The model under review builds one solid part; all positions refer to its coordinate system, in mm. A direction names the side the tool comes from. Give positions to 0.01 mm unless a question says otherwise; leave off trailing zeros. Order: outer loops, then holes, each group sorted by start corner. A loop starts at its lowest first (then second) coordinate and runs counter-clockwise, first axis right, second up.
```python
from build123d import *

# Parameters (mm, degrees)
BOSS_EXTRUDE1_DEPTH              = 5
FILLET1_R                        = 3
TAP_DRILL_FOR_M8X1_25_TAP1_D     = 6.8
TAP_DRILL_FOR_M8X1_25_TAP1_DEPTH = 8
TAP_DRILL_FOR_M8X1_25_TAP1_TIP   = 2.042926105


with BuildPart() as part:
    # Sketch1 → Boss-Extrude1 (new body)
    with BuildSketch(Plane(origin=(0, 0, 0), x_dir=(1, 0, 0), z_dir=(0, 1, 0))):
        with BuildLine():
            Line((32, 42), (-32, 42))
            ThreePointArc((-32, 42), (-39.071067812, 39.071067812), (-42, 32))
            Line((-42, 32), (-42, -32))
            ThreePointArc((-42, -32), (-39.071067812, -39.071067812), (-32, -42))
            Line((-32, -42), (32, -42))
            ThreePointArc((32, -42), (39.071067812, -39.071067812), (42, -32))
            Line((42, -32), (42, 32))
            ThreePointArc((42, 32), (39.071067812, 39.071067812), (32, 42))
        make_face()
    extrude(amount=BOSS_EXTRUDE1_DEPTH)

    # Sketch3 → Revolve2 (revolve)
    with BuildSketch(Plane.XY, mode=Mode.PRIVATE) as revolve2_sk:
        with BuildLine():
            Line((-21.830169384, 5), (-12.5, 5))
            Line((-12.5, 5), (-11.15, 5))
            Line((-11.15, 5), (-11.15, 12))
            Line((-11.15, 12), (-12.5, 12))
            ThreePointArc((-12.5, 12), (-16.03878275, 6.998773158), (-21.830169384, 5))
        make_face()
        with BuildLine():
            Line((-12.5, 12), (-11.15, 12))
            ThreePointArc((-11.15, 12), (-11.537197996, 13.009021804), (-12.5, 13.5))
            Line((-12.5, 13.5), (-15.5, 13.5))
            ThreePointArc((-15.5, 13.5), (-13.822949017, 13.104101966), (-12.5, 12))
        make_face()
    revolve(revolve2_sk.sketch.rotate(Axis((0, 0, 0), (0, -1, 0)), 270), axis=Axis((0, 0, 0), (0, -1, 0)))

    # Sketch3_5 → Cut-Revolve2 (revolve, cut)
    with BuildSketch(Plane.XY, mode=Mode.PRIVATE) as cut_revolve2_sk:
        with BuildLine():
            Line((0, 0), (0, 5))
            Line((0, 5), (-7.6, 5))
            ThreePointArc((-7.6, 5), (-8.694616444, 4.701278719), (-9.6, 4.017392631))
            Line((-9.6, 4.017392631), (-9.6, 0))
            Line((-9.6, 0), (0, 0))
        make_face()
    revolve(cut_revolve2_sk.sketch.rotate(Axis((0, 0, 0), (0, -1, 0)), 270), axis=Axis((0, 0, 0), (0, -1, 0)), mode=Mode.SUBTRACT)

    # Fillet1
    fillet1_edges = [part.edges().sort_by_distance(p)[0] for p in [
        (39.071067812, 5, 39.071067812),
        (0, 5, 42),
        (-39.071067812, 5, 39.071067812),
        (-42, 5, 0),
        (-39.071067812, 5, -39.071067812),
        (0, 5, -42),
        (39.071067812, 5, -39.071067812),
        (42, 5, 0),
    ]]
    fillet(fillet1_edges, radius=FILLET1_R)

    # Tap Drill for M8x1.25 Tap1
    with Locations(Plane(origin=(0, 5, 0), x_dir=(1, 0, 0), z_dir=(0, 1, 0))):
        with Locations((-32, 32), (-32, -32), (32, -32), (32, 32)):
            Hole(TAP_DRILL_FOR_M8X1_25_TAP1_D / 2, depth=TAP_DRILL_FOR_M8X1_25_TAP1_DEPTH)
            with Locations((0, 0, -(TAP_DRILL_FOR_M8X1_25_TAP1_DEPTH + TAP_DRILL_FOR_M8X1_25_TAP1_TIP / 2))):  # 118° drill point
                Cone(0, TAP_DRILL_FOR_M8X1_25_TAP1_D / 2, TAP_DRILL_FOR_M8X1_25_TAP1_TIP, mode=Mode.SUBTRACT)


solid = part.part
```
Item 1: Take a section at A-A (x = 0). Give the boundary of the cut face in (y, z), and give its area (3 significant figures).
Values found:
outline: (0, -42) - (2, -42) arc R3 ccw to (5, -39) - (5, -21.83) arc R10 cw to (12, -12.5) arc R3.75 cw to (13.5, -15.5) - (13.5, -12.5) arc R1.51 ccw to (12, -11.15) - (5, -11.15) - (5, -7.6) arc R3 cw to (4.02, -9.6) - (0, -9.6) - close; (0, 9.6) - (4.02, 9.6) arc R3 cw to (5, 7.6) - (5, 11.15) - (12, 11.15) arc R1.51 ccw to (13.5, 12.5) - (13.5, 15.5) arc R3.75 cw to (12, 12.5) arc R10 cw to (5, 21.83) - (5, 39) arc R3 ccw to (2, 42) - (0, 42) - close
area: 382 mm2
Item 2: For faces 1 (the cylindrical face through (-35.14, 2.46, 33.3)), 2 (the cylindrical face through (10.885, 8.549, -2.417)), 3 (the cylindrical face through (-8.095, 1.981, 5.161)), list the 3-axis set-ups (+Z, -Z, +X, -X, +Y, -Y) from which the entire face can be reached by the end or side of a thin tool; tool diameter is ignored.
Values found:
face 1: +Y, -Y
face 2: +Y
face 3: -Y
Item 3: Take a section at D-D (x = -24). Give the boundary of the cut face in (y, z).
Values found:
outline: (0, -42) - (2, -42) arc R3 ccw to (5, -39) - (5, 39) arc R3 ccw to (2, 42) - (0, 42) - close
Item 4: Take a section at C-C (z = 23.5). Give the boundary of the cut face in (x, y), and give its area (3 significant figures).
Values found:
outline: (-42, 0) - (42, 0) - (42, 2) arc R3 ccw to (39, 5) - (-39, 5) arc R3 ccw to (-42, 2) - close
area: 416 mm2
Item 5: Clearance check with flat-ended pins moving along their axes: pin 1 Ø6 at (x, z) = (32, -32) entering from -Y; pin 2 Ø6 at (y, z) = (7, 15) entering from +X; pin 3 Ø8 at (x, y) = (7, 3.5) entering from +Z; pin 4 Ø17.5 at (x, z) = (0, 0) entering from -Y. State where each tip first meets the part, or that it passes through.
Values found:
pin 1: passes through
pin 2: stops at x = 41.24
pin 3: stops at z = 42
pin 4: stops at y = 4.67
Item 6: For line 1 (Z direction, x = 32, y = 1.7); line 2 (X direction, y = 1.65, z = 0); line 3 (Z direction, x = 31, y = 4), list the stretches that pass through material, from the lowest coordinate up.
Values found:
line 1: z = -42 to -35.4, -28.6 to 28.6, 35.4 to 42
line 2: x = -42 to -9.6, 9.6 to 42
line 3: z = -41.24 to -35.25, -28.75 to 28.75, 35.25 to 41.24
Item 7: Take a section at B-B (z = 0). Give the boundary of the cut face in (x, y).
Values found:
outline: (-42, 0) - (-9.6, 0) - (-9.6, 4.02) arc R3 cw to (-7.6, 5) - (-11.15, 5) - (-11.15, 12) arc R1.51 ccw to (-12.5, 13.5) - (-15.5, 13.5) arc R3.75 cw to (-12.5, 12) arc R10 cw to (-21.83, 5) - (-39, 5) arc R3 ccw to (-42, 2) - close; (7.6, 5) arc R3 cw to (9.6, 4.02) - (9.6, 0) - (42, 0) - (42, 2) arc R3 ccw to (39, 5) - (21.83, 5) arc R10 cw to (12.5, 12) arc R3.75 cw to (15.5, 13.5) - (12.5, 13.5) arc R1.51 ccw to (11.15, 12) - (11.15, 5) - close
